For this review, take the finished solid that the model builds, in its own axes (mm). Face numbers are marked on the shaded views. A direction names the side the tool comes from. Round coordinates to 2 decimals unless told otherwise and drop trailing zeros. Write each loop counter-clockwise with the first axis right and the second up, starting at its lowest first coordinate (ties: lowest second). Pieces come first, ordered by that corner, then holes. Notation, with made-up numbers: (-8.75, -40) - (9.25, -40) arc R21 ccw to (9.25, -7) - close; hole circle Ø6 at (49.5, 89.25). An arc over 180 degrees is marked (long way). One line per item, written item: value. Start each with the question number.
Q1. For probe 1 along Y at (x, z) = (-107.95, -130.55) (3 decimals); probe 2 along Y at (x, z) = (107, -130); probe 3 along X at (y, z) = (176, -127), list the stretches that pass through material, from the lowest coordinate up.
Q2. Add section B-B on z = -117. Write out the cut boundary in (x, y), and give its area (3 significant figures).
Q3. Tool access review of the marked faces 1, 2 and 3: name each direction out of +Z, -Z, +X, -X, +Y, -Y from which nothing blocks a thin tool from reaching the whole face with its end or side.
Q4. Clearance check with flat-ended pins moving along their axes: pin 1 Ø7 at (x, y) = (-110.5, 85) entering from +Z; pin 2 Ø15.5 at (x, y) = (-107.95, 152.68) entering from -Z; pin 3 Ø1 at (y, z) = (22.5, -111.5) entering from -X; pin 4 Ø6 at (y, z) = (66.5, -111) entering from -X. State where each tip first meets the part, or that it passes through.
Q5. Add section A-A on y = 113.5. Write out the cut boundary in (x, z), and give its area (3 significant figures).
Q6. Mouldability with a two-part tool opening along X and no side actions: class the marked faces 4 and 5 as +X half, -X half, draft (parallel to the pull), parting line (faces both ways), or undercut.
Q7. Add section C-C on x = -53.5. Write out the cut boundary in (y, z).
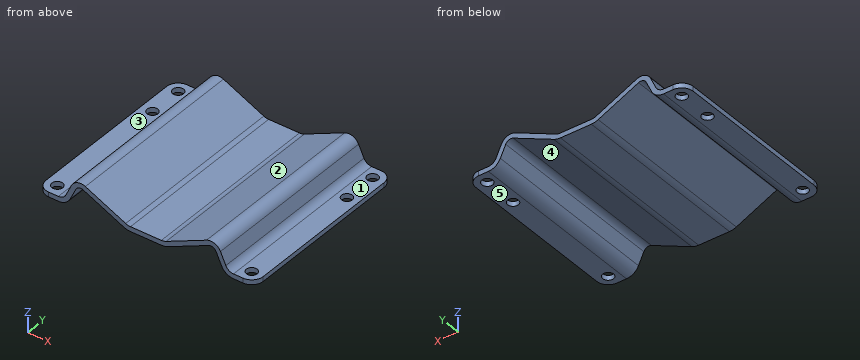
```python
from build123d import *

# Parameters (mm, degrees)
F1_DEPTH = 203.2
F2_R     = 5.9944
F3_DEPTH = 34.085578
F4_R     = 6.35
F5_R     = 11.6586
F6_R     = 12.7
F7_R     = 18.0086
F8_R     = 9.398
F9_R     = 14.7066
F10_R    = 12.7


with BuildPart() as f1:
    # F0 (on Front) → F1 (new body)
    with BuildSketch(Plane.XZ):
        Polygon((77.8321, -97.893822), (19.934749, -124.8918), (0, -124.8918), (-19.934749, -124.8918), (-77.8321, -97.893822), (-91.250559, -126.6698), (-120.65, -126.6698), (-120.65, -131.9784), (-87.868608, -131.9784), (-75.264386, -104.948559), (-21.111638, -130.2004), (0, -130.2004), (21.111638, -130.2004), (75.264386, -104.948559), (87.868608, -131.9784), (120.65, -131.9784), (120.65, -126.6698), (91.250559, -126.6698), align=None)
    extrude(amount=-F1_DEPTH)

    # F2 (on face) → F3 (cut, through all)
    with BuildSketch(Plane(origin=(0, 0, -131.9784), x_dir=(1, 0, 0), z_dir=(0, 0, -1))):
        with Locations((107.95, -12.7)):
            Circle(F2_R)
        with Locations((107.95, -152.6794)):
            Circle(F2_R)
        with Locations((107.95, -190.5)):
            Circle(F2_R)
        with Locations((-107.95, -190.5)):
            Circle(F2_R)
        with Locations((-107.95, -152.6794)):
            Circle(F2_R)
        with Locations((-107.95, -12.7)):
            Circle(F2_R)
    extrude(amount=-F3_DEPTH, mode=Mode.SUBTRACT)

    # F4
    f4_edges = [f1.edges().sort_by_distance(p)[0] for p in [
        (-75.264386, 101.6, -104.948559),
        (75.264386, 101.6, -104.948559),
    ]]
    fillet(f4_edges, radius=F4_R)

    # F5
    f5_edges = [f1.edges().sort_by_distance(p)[0] for p in [
        (77.8321, 101.6, -97.893822),
        (-77.8321, 101.6, -97.893822),
    ]]
    fillet(f5_edges, radius=F5_R)

    # F6
    f6_edges = [f1.edges().sort_by_distance(p)[0] for p in [
        (-19.934749, 101.6, -124.8918),
        (19.934749, 101.6, -124.8918),
    ]]
    fillet(f6_edges, radius=F6_R)

    # F7
    f7_edges = [f1.edges().sort_by_distance(p)[0] for p in [
        (-21.111638, 101.6, -130.2004),
        (21.111638, 101.6, -130.2004),
    ]]
    fillet(f7_edges, radius=F7_R)

    # F8
    f8_edges = [f1.edges().sort_by_distance(p)[0] for p in [
        (-91.250559, 101.6, -126.6698),
        (91.250559, 101.6, -126.6698),
    ]]
    fillet(f8_edges, radius=F8_R)

    # F9
    f9_edges = [f1.edges().sort_by_distance(p)[0] for p in [
        (-87.868608, 101.6, -131.9784),
        (87.868608, 101.6, -131.9784),
    ]]
    fillet(f9_edges, radius=F9_R)

    # F10
    f10_edges = [f1.edges().sort_by_distance(p)[0] for p in [
        (-120.65, 0, -129.3241),
        (120.65, 0, -129.3241),
        (-120.65, 203.2, -129.3241),
        (120.65, 203.2, -129.3241),
    ]]
    fillet(f10_edges, radius=F10_R)


solid = f1.part
```
Result set:
1. probe 1: y = 0 to 6.706, 18.694 to 146.685, 158.674 to 184.506, 196.494 to 203.2
1. probe 2: y = 0 to 6.78, 18.62 to 146.76, 158.6 to 184.58, 196.42 to 203.2
1. probe 3: x = -120.65 to -86.21, -27.97 to 27.97, 86.21 to 120.65
2. outline: (-86.74, 0) - (-80.88, 0) - (-80.88, 203.2) - (-86.74, 203.2) - close; (-49.42, 0) - (-36.86, 0) - (-36.86, 203.2) - (-49.42, 203.2) - close; (36.86, 0) - (49.42, 0) - (49.42, 203.2) - (36.86, 203.2) - close; (80.88, 0) - (86.74, 0) - (86.74, 203.2) - (80.88, 203.2) - close
2. area: 7,490 mm^2
3. face 1: +Z, +X, +Y, -Y
3. face 2: +Z, +Y, -Y
3. face 3: +Z, -X, +Y, -Y
4. pin 1: stops at z = -126.67
4. pin 2: stops at z = -131.98
4. pin 3: stops at x = -84.41
4. pin 4: stops at x = -85.34
5. outline: (-120.65, -131.98) - (-97.24, -131.98) arc R14.71 ccw to (-83.91, -123.49) - (-77.95, -110.7) arc R6.35 cw to (-69.51, -107.63) - (-24.73, -128.51) arc R18.01 ccw to (-17.12, -130.2) - (17.12, -130.2) arc R18.01 ccw to (24.73, -128.51) - (69.51, -107.63) arc R6.35 cw to (77.95, -110.7) - (83.91, -123.49) arc R14.71 ccw to (97.24, -131.98) - (120.65, -131.98) - (120.65, -126.67) - (97.24, -126.67) arc R9.4 cw to (88.72, -121.24) - (82.76, -108.46) arc R11.66 ccw to (67.27, -102.82) - (22.49, -123.7) arc R12.7 cw to (17.12, -124.89) - (-17.12, -124.89) arc R12.7 cw to (-22.49, -123.7) - (-67.27, -102.82) arc R11.66 ccw to (-82.76, -108.46) - (-88.72, -121.24) arc R9.4 cw to (-97.24, -126.67) - (-120.65, -126.67) - close
5. area: 1,470 mm^2
6. face 4: undercut
6. face 5: draft
7. outline: (0, -115.1) - (203.2, -115.1) - (203.2, -109.24) - (0, -109.24) - close
